Design review of the part shown in the three views and the two pictorial views. Dimensions are in mm from the part's minimum x, y and z. A direction names the side the tool comes from. Give positions to 0.01 mm unless a question says otherwise; leave off trailing zeros. Loops run counter-clockwise (first coordinate to the right, second up) from the corner with the lowest first, then second, coordinate; pieces in that order, holes last. Notation, with made-up numbers: (51, 9) - (76, 9) arc R5 ccw to (76, 13) - close; hole circle Ø3 at (56, -29.75). An arc over 180 degrees is marked (long way). Answer in a Markdown table with one row per item.
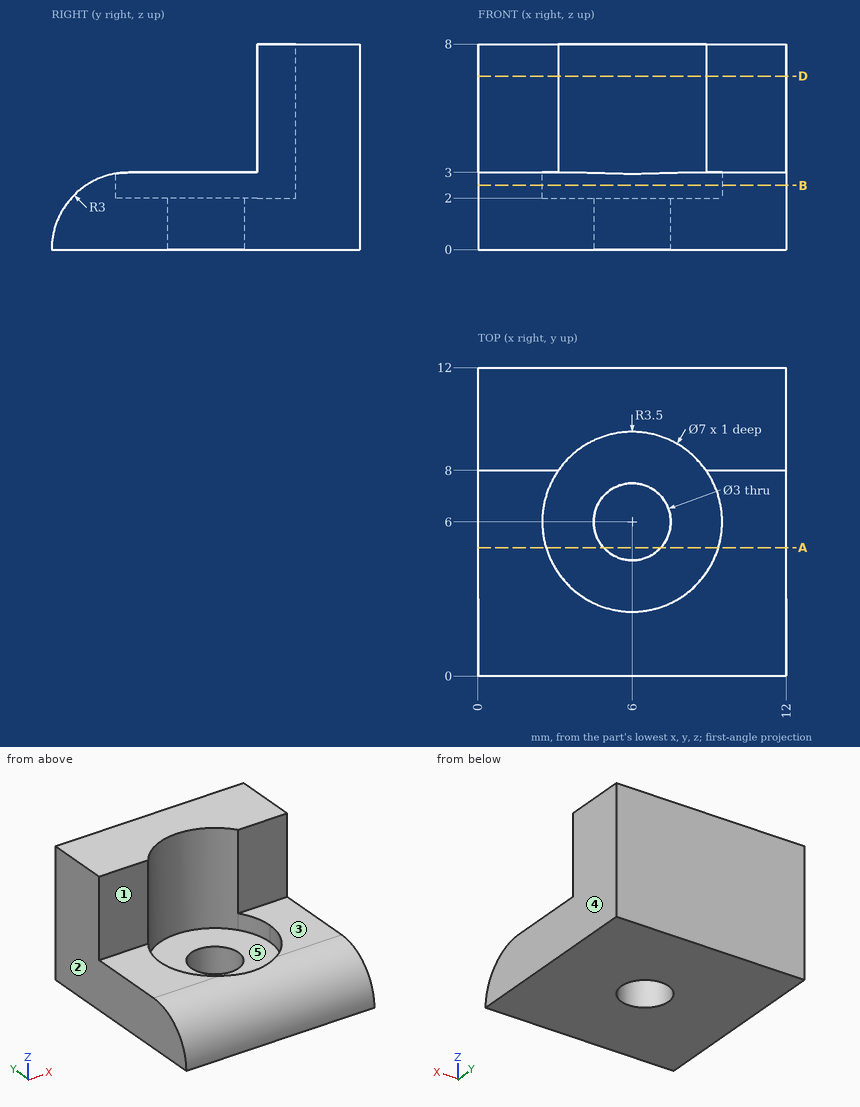
1. Wall thickness on line 1 (Z direction, x = 4, y = 4.25); line 2 (Y direction, x = 11.25, z = 6.5); line 3 (Y direction, x = 6, z = 3.5): over which ranges is each line inside the solid? List them lowest first. Write a range as [from, to].
Values:
| item | result |
|---|---|
| line 1 | z = [0, 2] |
| line 2 | y = [8, 12] |
| line 3 | y = [9.5, 12] |
2. We need section A-A, the plane y = 5. Give the boundary of the cut face in (x, z), and give its area (3 significant figures).
Values:
| item | result |
|---|---|
| outline | (0, 0) - (4.88, 0) - (4.88, 2) - (2.65, 2) - (2.65, 3) - (0, 3) - close; (7.12, 0) - (12, 0) - (12, 3) - (9.35, 3) - (9.35, 2) - (7.12, 2) - close |
| area | 24.8 mm^2 |
3. We need section D-D, the plane z = 6.75. Give the boundary of the cut face in (x, y), and give its area (3 significant figures).
Values:
| item | result |
|---|---|
| outline | (0, 8) - (3.13, 8) arc R3.5 cw to (8.87, 8) - (12, 8) - (12, 12) - (0, 12) - close |
| area | 42.0 mm^2 |
4. Clearance check with flat-ended pins moving along their axes: pin 1 (1 mm diameter, centred on x = 9, z = 4.5, fed in from -Y); pin 2 (4 mm diameter, centred on x = 6, z = 3, fed in from -Y); pin 3 (1.3 mm diameter, centred on x = 2.5, y = 6.5, fed in from +Z). State where each tip first meets the part, or that it passes through.
Values:
| item | result |
|---|---|
| pin 1 | stops at y = 8 |
| pin 2 | stops at y = 0.17 |
| pin 3 | stops at z = 3 |
5. We need section B-B, the plane z = 2.5. Give the boundary of the cut face in (x, y), and give its area (3 significant figures).
Values:
| item | result |
|---|---|
| outline | (0, 1.34) - (12, 1.34) - (12, 12) - (0, 12) - close; hole circle Ø7 at (6, 6) |
| area | 89.4 mm^2 |
6. For the marked faces 1 and 2, list the 3-axis set-ups (+Z, -Z, +X, -X, +Y, -Y) from which the entire face can be reached by the end or side of a thin tool; tool diameter is ignored.
Values:
| item | result |
|---|---|
| face 1 | +Z, +X, -X, -Y |
| face 2 | +Z, -Z, -X, +Y, -Y |
7. Mouldability with a two-part tool opening along X and no side actions: class the marked faces 3, 4 and 5 as released by +X, released by -X, zero draft, split by the parting line, or undercut.
Values:
| item | result |
|---|---|
| face 3 | zero draft |
| face 4 | released by +X |
| face 5 | undercut |
